Verification items for this drawing (mm, ordinates from the low corner). Round coordinates to 2 decimals unless told otherwise and drop trailing zeros. Loops run counter-clockwise (first coordinate to the right, second up) from the corner with the lowest first, then second, coordinate; pieces in that order, holes last. Notation, with made-up numbers: M 82,43 L 101,43 A25 ccw 101,65 Z; hole C 57.25,28 d9. An arc over 180 degrees is marked long. One line per item, written item: value.
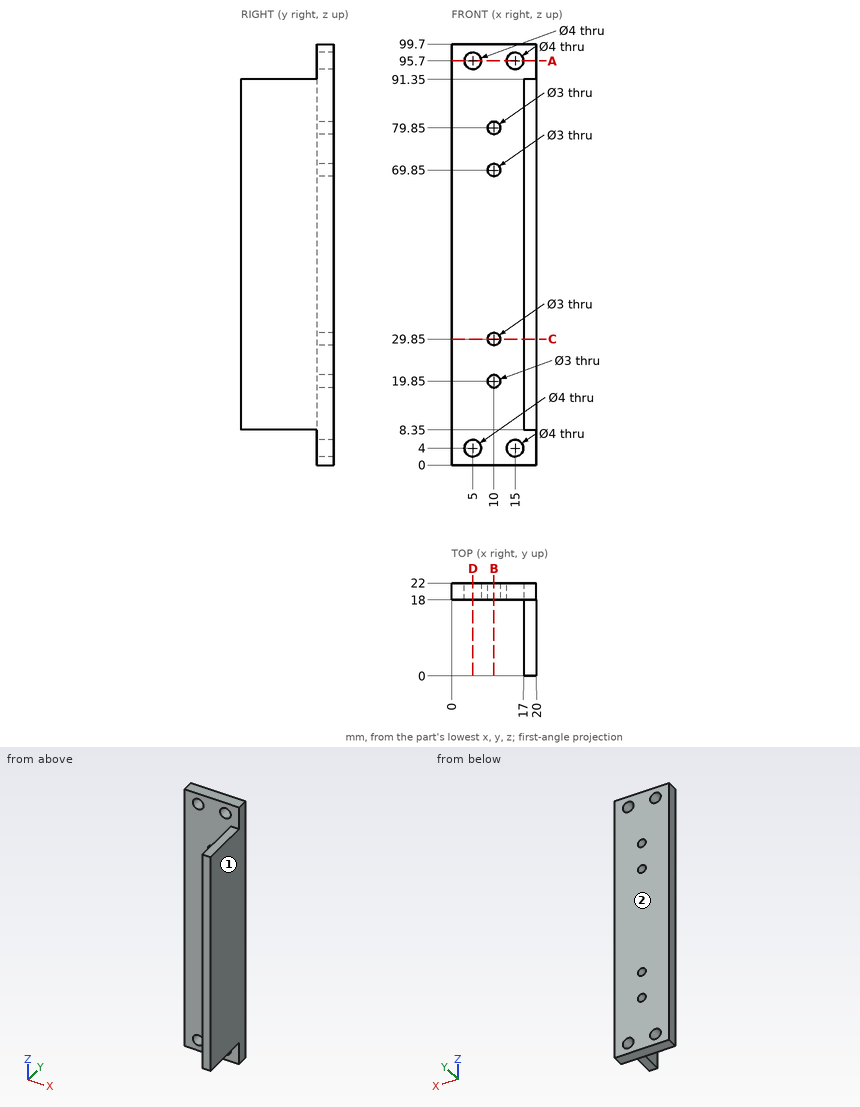
(1) Sectioned sample at D-D on x = 5. Enter the section's corners in (y, z).
Completed:
outline: M 18,0 L 22,0 L 22,2 L 18,2 Z; M 18,6 L 22,6 L 22,93.7 L 18,93.7 Z; M 18,97.7 L 22,97.7 L 22,99.7 L 18,99.7 Z
(2) Depth check by flat-ended pin: pin 1 Ø4 at (x, z) = (10, 69.85) entering from +Y; pin 2 Ø3.5 at (x, y) = (18.5, 6.5) entering from +Z; pin 3 Ø3 at (x, z) = (5.5, 34.5) entering from -Y; pin 4 Ø9 at (y, z) = (12, 47.5) entering from -X. Enter the tip coordinate at first touch or a pass-through.
Completed:
pin 1: stops at y = 22
pin 2: stops at z = 91.35
pin 3: stops at y = 18
pin 4: stops at x = 17
(3) Sectioned sample at A-A on z = 95.7. Enter the section's corners in (x, y), and give its area (3 significant figures).
Completed:
outline: M 0,18 L 3,18 L 3,22 L 0,22 Z; M 7,18 L 13,18 L 13,22 L 7,22 Z; M 17,18 L 20,18 L 20,22 L 17,22 Z
area: 48.0 mm^2
(4) Sectioned sample at B-B on x = 10. Enter the section's corners in (y, z), and give its area (3 significant figures).
Completed:
outline: M 18,0 L 22,0 L 22,18.35 L 18,18.35 Z; M 18,21.35 L 22,21.35 L 22,28.35 L 18,28.35 Z; M 18,31.35 L 22,31.35 L 22,68.35 L 18,68.35 Z; M 18,71.35 L 22,71.35 L 22,78.35 L 18,78.35 Z; M 18,81.35 L 22,81.35 L 22,99.7 L 18,99.7 Z
area: 351 mm^2
(5) Sectioned sample at C-C on z = 29.85. Enter the section's corners in (x, y).
Completed:
outline: M 0,18 L 8.5,18 L 8.5,22 L 0,22 Z; M 11.5,18 L 17,18 L 17,0 L 20,0 L 20,22 L 11.5,22 Z
(6) Thickness scan on L1, parallel to Z at x = 5, y = 21.25; L2, parallel to X at y = 19.25, z = 95.7; L3, parallel to Z at x = 10, y = 21.1. Record the ranges inside material, lowest first. Write a range as from..to.
Completed:
L1: z = 0..2, 6..93.7, 97.7..99.7
L2: x = 0..3, 7..13, 17..20
L3: z = 0..18.35, 21.35..28.35, 31.35..68.35, 71.35..78.35, 81.35..99.7
(7) Mould release check, pull along Y, two halves, no side actions. Record for the marked faces 1 and 2: +Y half, -Y half, draft (parallel to the pull), parting line (faces both ways), or undercut.
Completed:
face 1: draft
face 2: +Y half
